Input: dimensioned drawing with shaded views. Units: mm. Origin: part minimum x, y, z. A direction names the side the tool comes from. Round coordinates to 2 decimals unless told otherwise and drop trailing zeros. Loops run counter-clockwise (first coordinate to the right, second up) from the corner with the lowest first, then second, coordinate; pieces in that order, holes last. Notation, with made-up numbers: (42.25, 54) - (94.25, 54) arc R9 ccw to (94.25, 67) - close; hole circle Ø9 at (42.25, -8.5). An arc over 180 degrees is marked (long way). Answer as a JSON object with one key per item and string values. Group by question number.
Item 1: Draft query along Z for the marked faces 3, 4 and 5. Return one class per face: released by +Z, released by -Z, zero draft, split by the parting line, or undercut.
Item 2: Section B-B (z = 7). Return the cut outline in (x, y).
Item 3: Section D-D (x = 2.25). Return the cut outline in (y, z).
Item 4: Reachability of the marked faces 1 and 2 from +Z, -Z, +X, -X, +Y, -Y: full face, straight path, thin tool, end or side. Return the list, or none.
Item 5: Section A-A (x = 6). Return the cut outline in (y, z), plus the area to 3 significant figures.
Item 6: First-contact query: pin 1 (1 mm diameter, centred on x = 7, z = 7, fed in from -Y); pin 2 (2 mm diameter, centred on x = 10.5, y = 16, fed in from +Z). Flat tips, straight axial feed; report the tip coordinate or a pass-through.
Item 7: Section C-C (y = 14.75). Return the cut outline in (x, z), plus the area to 3 significant figures.
Item 8: Line query: line 1 (X direction, y = 11, z = 8.75); line 2 (X direction, y = 6, z = 7); line 3 (Z direction, x = 3.75, y = 4). Output: solid intervals per line, ascending.
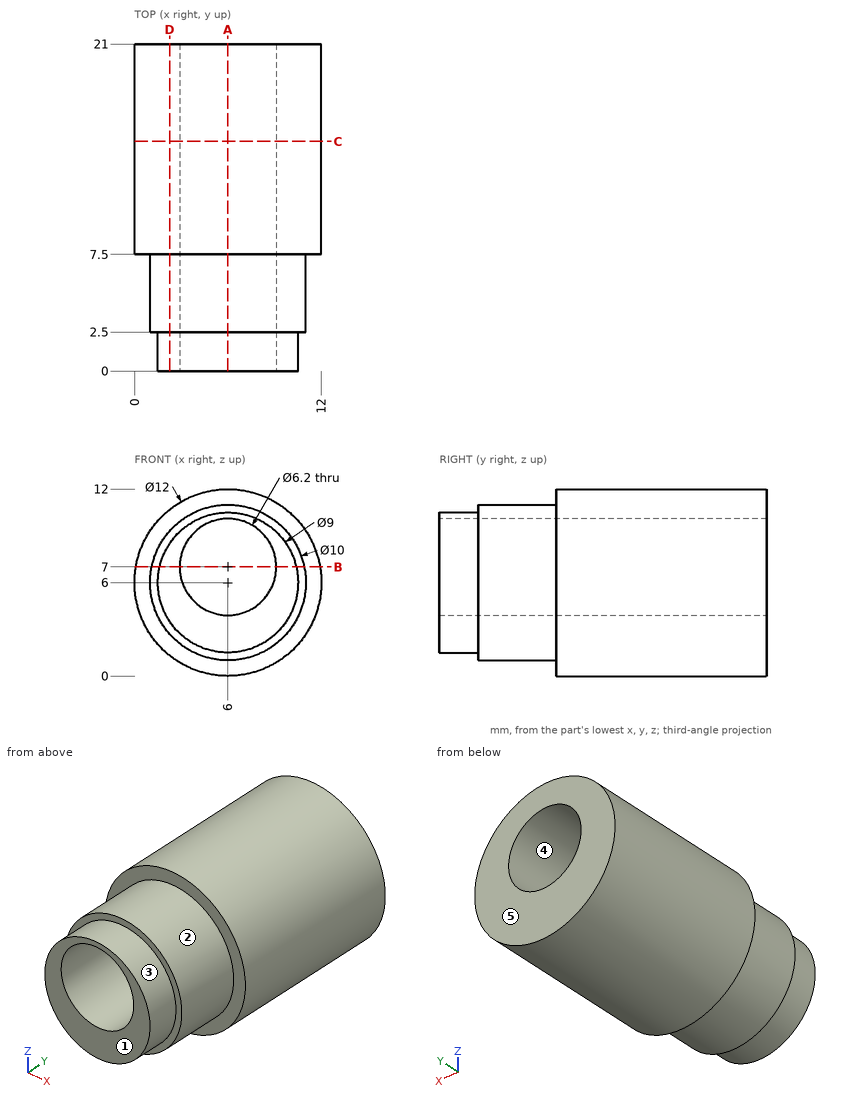
Values:
{
 "1": {"face 3": "split by the parting line", "face 4": "undercut", "face 5": "zero draft"},
 "2": {"outline": "(0.08, 7.5) - (1.1, 7.5) - (1.1, 2.5) - (1.61, 2.5) - (1.61, 0) - (2.9, 0) - (2.9, 21) - (0.08, 21) - close; (9.1, 0) - (10.39, 0) - (10.39, 2.5) - (10.9, 2.5) - (10.9, 7.5) - (11.92, 7.5) - (11.92, 21) - (9.1, 21) - close"},
 "3": {"outline": "(0, 3.51) - (2.5, 3.51) - (2.5, 2.69) - (7.5, 2.69) - (7.5, 1.32) - (21, 1.32) - (21, 10.68) - (7.5, 10.68) - (7.5, 9.31) - (2.5, 9.31) - (2.5, 8.49) - (0, 8.49) - close"},
 "4": {"face 1": "+Z, -Z, +X, -X, -Y", "face 2": "-Y"},
 "5": {"outline": "(0, 1.5) - (2.5, 1.5) - (2.5, 1) - (7.5, 1) - (7.5, 0) - (21, 0) - (21, 3.9) - (0, 3.9) - close; (0, 10.1) - (21, 10.1) - (21, 12) - (7.5, 12) - (7.5, 11) - (2.5, 11) - (2.5, 10.5) - (0, 10.5) - close", "area": "104 mm^2"},
 "6": {"pin 1": "passes through", "pin 2": "stops at z = 10.87"},
 "7": {"outline": "circle Ø12 at (6, 6); hole circle Ø6.2 at (6, 7)", "area": "82.9 mm^2"},
 "8": {"line 1": "x = 0.67 to 3.44, 8.56 to 11.33", "line 2": "x = 1.1 to 2.9, 9.1 to 10.9", "line 3": "z = 1.53 to 4.87, 9.13 to 10.47"}
}
